Part model, mm, in its own coordinate system. Face numbers are marked on the shaded views. A direction names the side the tool comes from. Round coordinates to 2 decimals unless told otherwise and drop trailing zeros. Loops run counter-clockwise (first coordinate to the right, second up) from the corner with the lowest first, then second, coordinate; pieces in that order, holes last.
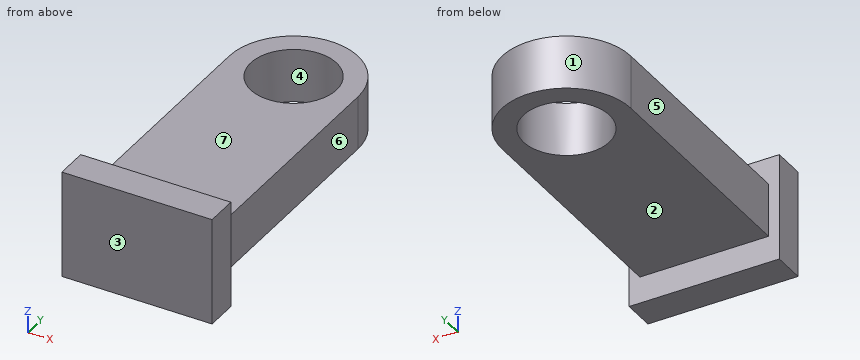
from build123d import *

# Parameters (mm, degrees)
SKETCH1_R               = 6
SKETCH1_R_2             = 4
BOSS_EXTRUDE1_DEPTH     = 5
SKETCH2_W               = 12
SKETCH2_H               = 5
BOSS_EXTRUDE2_DEPTH     = 22
CUT_EXTRUDE1_DEPTH      = 24.34523506
CUT_EXTRUDE1_DEPTH_BACK = 24.34523506
SKETCH5_R               = 4
SKETCH6_W               = 14
SKETCH6_H               = 10
BOSS_EXTRUDE3_DEPTH     = 3


with BuildPart() as part:
    # Sketch1 → Boss-Extrude1 (new body)
    with BuildSketch(Plane.XY):
        Circle(SKETCH1_R)
        Circle(SKETCH1_R_2, mode=Mode.SUBTRACT)
    extrude(amount=BOSS_EXTRUDE1_DEPTH)

    # Sketch2 → Boss-Extrude2 (add)
    with BuildSketch(Plane(origin=(0, 0, 0), x_dir=(1, 0, 0), z_dir=(0, 1, 0))):
        with Locations((0, -2.5)):
            Rectangle(SKETCH2_W, SKETCH2_H)
    extrude(amount=-BOSS_EXTRUDE2_DEPTH)

    # Sketch5 → Cut-Extrude1 (cut, two sides: drawn at the far end of the back side and taken through both)
    with BuildSketch(Plane.XY.offset(5).offset(-CUT_EXTRUDE1_DEPTH_BACK)):
        Circle(SKETCH5_R)
    extrude(amount=CUT_EXTRUDE1_DEPTH + CUT_EXTRUDE1_DEPTH_BACK, mode=Mode.SUBTRACT)

    # Sketch6 → Boss-Extrude3 (add)
    with BuildSketch(Plane.XZ.offset(22)):
        with Locations((0, 2.5)):
            Rectangle(SKETCH6_W, SKETCH6_H)
    extrude(amount=BOSS_EXTRUDE3_DEPTH)


solid = part.part
1) Slice it at B-B, the plane z = 4.5. Give the cut face in (x, y), then the cut area to 3 significant figures.
Values:
outline: (-7, -25) - (7, -25) - (7, -22) - (6, -22) - (6, 0) arc R6 ccw to (-6, 0) - (-6, -22) - (-7, -22) - close; hole circle Ø8 at (0, 0)
area: 312 mm2
2) Slice it at A-A, the plane x = 0. Give the cut face in (y, z), then the cut area to 3 significant figures.
Values:
outline: (-25, -2.5) - (-22, -2.5) - (-22, 0) - (-4, 0) - (-4, 5) - (-22, 5) - (-22, 7.5) - (-25, 7.5) - close; (4, 0) - (6, 0) - (6, 5) - (4, 5) - close
area: 130 mm2
3) Slice it at C-C, the plane y = 1.5. Give the cut face in (x, z).
Values:
outline: (-5.81, 0) - (-3.71, 0) - (-3.71, 5) - (-5.81, 5) - close; (3.71, 0) - (5.81, 0) - (5.81, 5) - (3.71, 5) - close
4) Wall check: line 1 along X through (y, z) = (0, 1.85); line 2 along Y through (x, z) = (0, 2.2); line 3 along Y through (x, z) = (2.5, 7.25). Give the ranges that are in metal, low to high.
Values:
line 1: x = -6 to -4, 4 to 6
line 2: y = -25 to -4, 4 to 6
line 3: y = -25 to -22
5) Mould opens along Y. For the marked faces 1, 2, 3 and 4 say: released by +Y, released by -Y, zero draft, split by the parting line, or undercut.
Values:
face 1: released by +Y
face 2: zero draft
face 3: released by -Y
face 4: undercut
6) Drop flat-ended pins along their axis: pin 1 Ø6.5 at (x, y) = (0, 0) entering from -Z; pin 2 Ø1 at (y, z) = (-3.5, 2.5) entering from -X; pin 3 Ø6 at (y, z) = (-5.5, -1) entering from +X; pin 4 Ø2 at (x, y) = (-2, -11.5) entering from +Z. Give the stop position or say it passes through.
Values:
pin 1: passes through
pin 2: stops at x = -6
pin 3: stops at x = 6
pin 4: stops at z = 5
7) Slice it at D-D, the plane z = 6.5. Give the cut face in (x, y), then the cut area to 3 significant figures.
Values:
outline: (-7, -25) - (7, -25) - (7, -22) - (-7, -22) - close
area: 42.0 mm2
8) Tool access for the marked faces 5, 6 and 7: list every direction of +Z, -Z, +X, -X, +Y, -Y with a clear straight run to the whole face (end or side of a thin tool).
Values:
face 5: +Z, -Z, -X, +Y
face 6: +Z, -Z, +X, +Y
face 7: +Z, +X, -X, +Y
